Here's the drawing with two shaded views (mm, measured from the low corner). I have some questions. Give positions to 0.01 mm unless a question says otherwise; leave off trailing zeros. Loops run counter-clockwise (first coordinate to the right, second up) from the corner with the lowest first, then second, coordinate; pieces in that order, holes last. Notation, with made-up numbers: (43.5, -37) -> (82.5, -37) arc R30 cw to (82.5, 0) -> close; hole circle Ø3 at (42, 66.25). An arc over 180 degrees is marked (long way). Put each result on its own line as item: value.
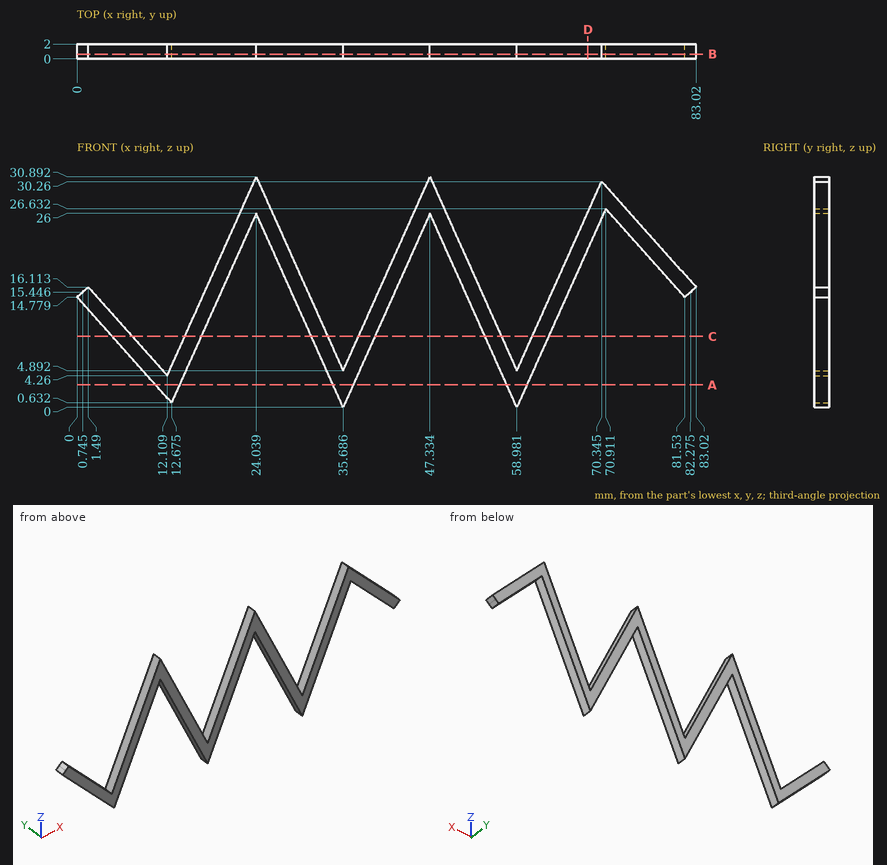
1. If we section it at C-C (z = 9.5): Count the separate pieces of the cut face and the enclosed holes in it.
Recorded:
separate pieces: 6
enclosed holes: 0
2. If we section it at D-D (x = 68.5): List the corners of the cut face in (y, z) for me.
Recorded:
outline: (0, 21.25) -> (2, 21.25) -> (2, 26.14) -> (0, 26.14) -> close
3. If we section it at A-A (z = 3): List the corners of the cut face in (x, y) for me (1 decimal), then the cut area to 3 significant figures.
Recorded:
outline: (10.6, 0) -> (13.7, 0) -> (13.7, 2) -> (10.6, 2) -> close; (34.3, 0) -> (37, 0) -> (37, 2) -> (34.3, 2) -> close; (57.6, 0) -> (60.3, 0) -> (60.3, 2) -> (57.6, 2) -> close
area: 17.1 mm^2
4. If we section it at B-B (y = 0.65): List the corners of the cut face in (x, z) for me (1 decimal).
Recorded:
outline: (0, 14.8) -> (12.7, 0.6) -> (24, 26) -> (35.7, 0) -> (47.3, 26) -> (59, 0) -> (70.9, 26.6) -> (81.5, 14.8) -> (83, 16.1) -> (70.3, 30.3) -> (59, 4.9) -> (47.3, 30.9) -> (35.7, 4.9) -> (24, 30.9) -> (12.1, 4.3) -> (1.5, 16.1) -> close
5. I need wall thicknesses on line 1 (X direction, y = 1.45, z = 27) (1 decimal); line 2 (X direction, y = 1.3, z = 1) (1 decimal); line 3 (X direction, y = 0.4, z = 20.5) (1 decimal). Which ranges of each line are inside material? Lowest first, please.
Recorded:
line 1: x = 22.3 to 25.8, 45.6 to 49.1, 68.9 to 73.3
line 2: x = 12.3 to 12.8, 35.2 to 36.1, 58.5 to 59.4
line 3: x = 19.4 to 21.6, 26.5 to 28.7, 42.7 to 44.9, 49.8 to 52, 66 to 68.2, 76.4 to 79.1
